The model under review builds one solid part; all positions refer to its coordinate system, in mm. Give positions to 0.01 mm unless a question says otherwise; leave off trailing zeros. Order: outer loops, then holes, each group sorted by start corner. A loop starts at its lowest first (then second) coordinate and runs counter-clockwise, first axis right, second up. Notation, with made-up numbers: (22, 62) - (48, 62) arc R29 ccw to (48, 89) - close; hole circle Ø5 at (80, -20.75). An arc over 180 degrees is marked (long way). Use CSV: the item, a comma, the result in double quotes. Start each with the question number.
1. Draft analysis for pull direction Z (two halves, no side actions). For faces 1 (the flat face through (-3, 17, 30)), 2 (the flat face through (-200, 17, 0)), 3 (the cylindrical face through (143.166, 17.745, -1.517)), 4 (the flat face through (-3, 17, -30)), state which applies: released by +Z, released by -Z, zero draft, split by the parting line, or undercut.
2. Take a section at B-B, the plane y = 6. Count the separate pieces of the cut face and the enclosed holes in it, then the cut area to 3 significant figures.
3. For pin 1 (4.5 mm diameter, centred on x = -168.77, z = -18.77, fed in from -Y); pin 2 (6 mm diameter, centred on x = -131.23, z = -18.77, fed in from -Y), all flat-tipped, find the tip position at first contact; note any pin that passes through.
4. To check wall thickness, follow line 1 (X direction, y = 20, z = 0); line 2 (X direction, y = 9.25, z = -18.77); line 3 (Z direction, x = 131.23, y = 7.25). State the ranges of each line that lie inside material, in increasing order. Write a range as [from, to].
5. Take a section at C-C, the plane x = -150. State the section outline as (y, z) points, then the cut area to 3 significant figures.
6. Take a section at A-A, the plane z = 0. State the section outline as (x, y) points, then the cut area to 3 significant figures.
```python
from build123d import *

# Parameters (mm, degrees)
SKETCH1_W                         = 400
SKETCH1_H                         = 60
BOSS_EXTRUDE1_DEPTH               = 35
SKETCH2_R                         = 7
CUT_EXTRUDE1_DEPTH                = 206.243757518
F_1_4_20_TAPPED_HOLE1_D           = 5.1054
F_1_4_20_TAPPED_HOLE1_DEPTH       = 18
F_1_4_20_TAPPED_HOLE1_CSINK_D     = 7.62
F_1_4_20_TAPPED_HOLE1_CSINK_ANGLE = 90
F_1_4_20_TAPPED_HOLE1_TIP         = 1.533816902


with BuildPart() as part:
    # Sketch1 → Boss-Extrude1 (new body)
    with BuildSketch(Plane(origin=(0, 0, 0), x_dir=(1, 0, 0), z_dir=(0, 1, 0))):
        Rectangle(SKETCH1_W, SKETCH1_H)
    extrude(amount=BOSS_EXTRUDE1_DEPTH)

    # Sketch2 → Cut-Extrude1 (cut, through all)
    with BuildSketch(Plane(origin=(0, 35, 0), x_dir=(1, 0, 0), z_dir=(0, 1, 0))):
        with Locations(Location((-150, 0, 0), (0, 0, 270))):
            Circle(SKETCH2_R)
        with Locations(Location((150, 0, 0), (0, 0, 270))):
            Circle(SKETCH2_R)
    extrude(amount=-CUT_EXTRUDE1_DEPTH, mode=Mode.SUBTRACT)

    # 1/4-20 Tapped Hole1
    with Locations(Plane.XZ):
        with Locations((-168.77, 18.77), (-131.23, 18.77), (-131.23, -18.77), (-168.77, -18.77), (131.23, 18.77), (168.77, 18.77), (168.77, -18.77), (131.23, -18.77)):
            CounterSinkHole(F_1_4_20_TAPPED_HOLE1_D / 2, F_1_4_20_TAPPED_HOLE1_CSINK_D / 2, depth=F_1_4_20_TAPPED_HOLE1_DEPTH, counter_sink_angle=F_1_4_20_TAPPED_HOLE1_CSINK_ANGLE)
            with Locations((0, 0, -(F_1_4_20_TAPPED_HOLE1_DEPTH + F_1_4_20_TAPPED_HOLE1_TIP / 2))):  # 118° drill point
                Cone(0, F_1_4_20_TAPPED_HOLE1_D / 2, F_1_4_20_TAPPED_HOLE1_TIP, mode=Mode.SUBTRACT)


solid = part.part
```
Determined:
1,face 1,"released by +Z"
1,face 2,"zero draft"
1,face 3,"undercut"
1,face 4,"released by -Z"
2,separate pieces,"1"
2,enclosed holes,"10"
2,area,"23,500 mm²"
3,pin 1,"stops at y = 18.18"
3,pin 2,"stops at y = 0.81"
4,line 1,"x = [-200, -157], [-143, 143], [157, 200]"
4,line 2,"x = [-200, -171.32], [-166.22, -133.78], [-128.68, 128.68], [133.78, 166.22], [171.32, 200]"
4,line 3,"z = [-30, -21.32], [-16.22, 16.22], [21.32, 30]"
5,outline,"(0, -30) - (35, -30) - (35, -7) - (0, -7) - close; (0, 7) - (35, 7) - (35, 30) - (0, 30) - close"
5,area,"1,610 mm²"
6,outline,"(-200, 0) - (-157, 0) - (-157, 35) - (-200, 35) - close; (-143, 0) - (143, 0) - (143, 35) - (-143, 35) - close; (157, 0) - (200, 0) - (200, 35) - (157, 35) - close"
6,area,"13,000 mm²"
